Model file for the job. Use its own axes, mm. A direction names the side the tool comes from. Round coordinates to 2 decimals unless told otherwise and drop trailing zeros. Order: outer loops, then holes, each group sorted by start corner. A loop starts at its lowest first (then second) coordinate and runs counter-clockwise, first axis right, second up. Notation, with made-up numbers: (-25, -7.5) -> (-18, -7.5) arc R21 cw to (-18, 31.5) -> close; hole circle Ø2 at (5, 54). An arc over 180 degrees is marked (long way). Use CSV: the item, a comma, the result in double quotes.
```python
from build123d import *

# Parameters (mm, degrees)
F0_W     = 90.7
F0_H     = 132
F0_W_2   = 82.7
F0_H_2   = 116
F0_W_3   = 71.7
F0_H_3   = 24
F1_DEPTH = 3


with BuildPart() as f1:
    # F0 (on Top) → F1 (new body)
    with BuildSketch(Plane.XY):
        with Locations((41.35, 59)):
            Rectangle(F0_W, F0_H)
        with Locations((41.35, 58)):
            Rectangle(F0_W_2, F0_H_2, mode=Mode.SUBTRACT)
        with Locations((41.35, 58)):
            Rectangle(F0_W_2, F0_H_2)
        with Locations((41.35, 72.25)):
            Rectangle(F0_W_3, F0_H_3, mode=Mode.SUBTRACT)
    extrude(amount=F1_DEPTH)


solid = f1.part
```
Q1. Cut at B-B (z = 2). Give the cut face in (x, y), plus the area to 3 significant figures.
From the geometry:
outline,"(-4, -7) -> (86.7, -7) -> (86.7, 125) -> (-4, 125) -> close; hole (5.5, 60.25) -> (77.2, 60.25) -> (77.2, 84.25) -> (5.5, 84.25) -> close"
area,"10,300 mm²"
Q2. Mould opens along Y. For faces 3 (the flat face through (-4, 58, 1)), 4 (the flat face through (41, 60.25, 1)), 5 (the flat face through (41, 125, 1)) say: +Y half, -Y half, draft (parallel to the pull), parting line (faces both ways), or undercut.
From the geometry:
face 3,"draft"
face 4,"undercut"
face 5,"+Y half"
Q3. Cut at A-A (x = 41.5). Give the cut face in (y, z), plus the area to 3 significant figures.
From the geometry:
outline,"(-7, 0) -> (60.25, 0) -> (60.25, 3) -> (-7, 3) -> close; (84.25, 0) -> (125, 0) -> (125, 3) -> (84.25, 3) -> close"
area,"324 mm²"
Q4. Which spindle directions (+Z, -Z, +X, -X, +Y, -Y) get a long thin tool onto all of the face, cutting with end or side? Do faces 1 (the flat face through (41, 84.25, 1)), 2 (the flat face through (41, 60, 0)). Say none if no direction does.
From the geometry:
face 1,"+Z, -Z"
face 2,"-Z, +X, -X, +Y, -Y"
Q5. Probe line 1 along Y through (x, z) = (58, 1.3); line 2 along X through (y, z) = (79, 1.9). List the from-to ranges inside material, lowest first.
From the geometry:
line 1,"y = -7 to 60.25, 84.25 to 125"
line 2,"x = -4 to 5.5, 77.2 to 86.7"
